Check sheet for the modelled part. Datum: model origin and axes. Units: mm. Coordinates: 2 decimals unless noted, no trailing zeros. Use a Markdown table: item, result. Add a question column.
1) Thickness scan on line 1 (Y direction, x = -32, z = 1.65); line 2 (Y direction, x = 57, z = 1.8); line 3 (Y direction, x = 352, z = 2.8). Record the ranges inside material, lowest first.
2) Sectioned sample at A-A, the plane z = 1.95. State how many separate pieces and enclosed holes the cut face has, then the cut area to 3 significant figures.
3) Go/stop test with a flat-tipped pin: P1, Ø8, axis at x = 210, y = -6.5, coming from the -Z side. Record where the tip stops, or that it passes through.
from build123d import *

# Parameters (mm, degrees)
SKETCH_1_W      = 526
SKETCH_1_H      = 78
SKETCH_1_R      = 10.25
SKETCH_1_R_2    = 2
EXTRUDE_1_DEPTH = 4


with BuildPart() as part:
    # Sketch 1 → Extrude 1 (new body)
    with BuildSketch(Plane.XY):
        with Locations((225, 0)):
            Rectangle(SKETCH_1_W, SKETCH_1_H)
        Circle(SKETCH_1_R, mode=Mode.SUBTRACT)
        with Locations((0, -19)):
            Circle(SKETCH_1_R_2, mode=Mode.SUBTRACT)
        with Locations((-13.435028843, -13.435028843)):
            Circle(SKETCH_1_R_2, mode=Mode.SUBTRACT)
        with Locations((-19, 0)):
            Circle(SKETCH_1_R_2, mode=Mode.SUBTRACT)
        with Locations((-13.435028843, 13.435028843)):
            Circle(SKETCH_1_R_2, mode=Mode.SUBTRACT)
        with Locations((0, 19)):
            Circle(SKETCH_1_R_2, mode=Mode.SUBTRACT)
        with Locations((13.435028843, 13.435028843)):
            Circle(SKETCH_1_R_2, mode=Mode.SUBTRACT)
        with Locations((19, 0)):
            Circle(SKETCH_1_R_2, mode=Mode.SUBTRACT)
        with Locations((13.435028843, -13.435028843)):
            Circle(SKETCH_1_R_2, mode=Mode.SUBTRACT)
        with Locations((450, -19)):
            Circle(SKETCH_1_R_2, mode=Mode.SUBTRACT)
        with Locations((450, 0)):
            Circle(SKETCH_1_R, mode=Mode.SUBTRACT)
        with Locations((436.564971157, -13.435028843)):
            Circle(SKETCH_1_R_2, mode=Mode.SUBTRACT)
        with Locations((431, 0)):
            Circle(SKETCH_1_R_2, mode=Mode.SUBTRACT)
        with Locations((436.564971157, 13.435028843)):
            Circle(SKETCH_1_R_2, mode=Mode.SUBTRACT)
        with Locations((450, 19)):
            Circle(SKETCH_1_R_2, mode=Mode.SUBTRACT)
        with Locations((463.435028843, 13.435028843)):
            Circle(SKETCH_1_R_2, mode=Mode.SUBTRACT)
        with Locations((469, 0)):
            Circle(SKETCH_1_R_2, mode=Mode.SUBTRACT)
        with Locations((463.435028843, -13.435028843)):
            Circle(SKETCH_1_R_2, mode=Mode.SUBTRACT)
        with Locations((-32, 33)):
            Circle(SKETCH_1_R_2, mode=Mode.SUBTRACT)
        with Locations((32, 33)):
            Circle(SKETCH_1_R_2, mode=Mode.SUBTRACT)
        with Locations((96, 33)):
            Circle(SKETCH_1_R_2, mode=Mode.SUBTRACT)
        with Locations((160, 33)):
            Circle(SKETCH_1_R_2, mode=Mode.SUBTRACT)
        with Locations((224, 33)):
            Circle(SKETCH_1_R_2, mode=Mode.SUBTRACT)
        with Locations((288, 33)):
            Circle(SKETCH_1_R_2, mode=Mode.SUBTRACT)
        with Locations((352, 33)):
            Circle(SKETCH_1_R_2, mode=Mode.SUBTRACT)
        with Locations((416, 33)):
            Circle(SKETCH_1_R_2, mode=Mode.SUBTRACT)
        with Locations((480, 33)):
            Circle(SKETCH_1_R_2, mode=Mode.SUBTRACT)
        with Locations((32, -33)):
            Circle(SKETCH_1_R_2, mode=Mode.SUBTRACT)
        with Locations((96, -33)):
            Circle(SKETCH_1_R_2, mode=Mode.SUBTRACT)
        with Locations((160, -33)):
            Circle(SKETCH_1_R_2, mode=Mode.SUBTRACT)
        with Locations((224, -33)):
            Circle(SKETCH_1_R_2, mode=Mode.SUBTRACT)
        with Locations((288, -33)):
            Circle(SKETCH_1_R_2, mode=Mode.SUBTRACT)
        with Locations((352, -33)):
            Circle(SKETCH_1_R_2, mode=Mode.SUBTRACT)
        with Locations((416, -33)):
            Circle(SKETCH_1_R_2, mode=Mode.SUBTRACT)
        with Locations((480, -33)):
            Circle(SKETCH_1_R_2, mode=Mode.SUBTRACT)
        with Locations((-32, -33)):
            Circle(SKETCH_1_R_2, mode=Mode.SUBTRACT)
        Polygon((40, 25), (92.613968548, 25), (141.098817033, -25), (40, -25), align=None, mode=Mode.SUBTRACT)
        Polygon((306.901182967, -25), (355.386031452, 25), (408, 25), (408, -25), align=None, mode=Mode.SUBTRACT)
        Polygon((284.613968548, -25), (232, -25), (232, 25), (333.098817033, 25), align=None, mode=Mode.SUBTRACT)
        Polygon((114.901182967, 25), (163.386031452, -25), (216, -25), (216, 25), align=None, mode=Mode.SUBTRACT)
    extrude(amount=EXTRUDE_1_DEPTH)


solid = part.part
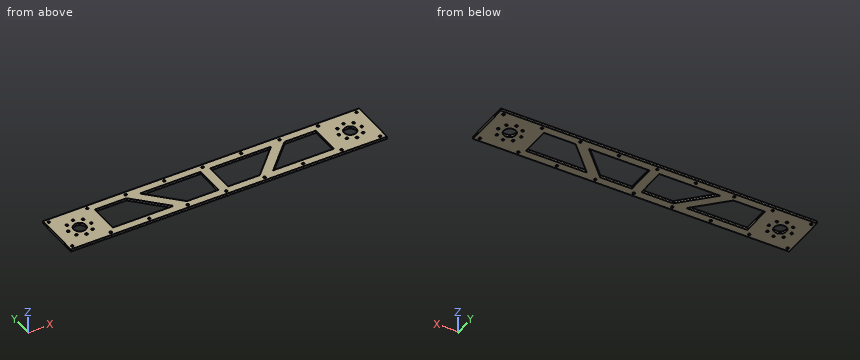
Solved:
| question | item | result |
|---|---|---|
| 1 | line 1 | y = -39 to -35, -31 to 31, 35 to 39 |
| 1 | line 2 | y = -39 to -25, 25 to 39 |
| 1 | line 3 | y = -39 to -35, -31 to -25, 21.51 to 31, 35 to 39 |
| 2 | separate pieces | 1 |
| 2 | enclosed holes | 40 |
| 2 | area | 24,600 mm2 |
| 3 | P1 | passes through |
